For this review, take the finished solid that the model builds, in its own axes (mm). Face numbers are marked on the shaded views. A direction names the side the tool comes from. Round coordinates to 2 decimals unless told otherwise and drop trailing zeros. Loops run counter-clockwise (first coordinate to the right, second up) from the corner with the lowest first, then second, coordinate; pieces in that order, holes last.
1. Clearance check with flat-ended pins moving along their axes: pin 1 Ø4 at (y, z) = (1, 4.5) entering from +X; pin 2 Ø17.5 at (x, z) = (4.5, -0.5) entering from +Y; pin 3 Ø3 at (y, z) = (4, 12) entering from -X. State where each tip first meets the part, or that it passes through.
2. Consider section B-B on z = 0. State the section outline as (x, y) points.
3. To check wall thickness, follow line 1 along Z through (x, y) = (-1.5, 6.75); line 2 along X through (y, z) = (6.5, 6.5); line 3 along X through (y, z) = (7, 6). State the ranges of each line that lie inside material, in increasing order.
4. Consider section C-C on x = 8. State the section outline as (y, z) points, then the cut area to 3 significant figures.
5. Consider section D-D on z = 7.5. State the section outline as (x, y) points.
6. Tool access review of the marked faces 4 and 5: name each direction out of +Z, -Z, +X, -X, +Y, -Y from which nothing blocks a thin tool from reaching the whole face with its end or side.
7. Draft analysis for pull direction Z (two halves, no side actions). For the marked faces 1, 2 and 3, state which applies: released by +Z, released by -Z, zero draft, split by the parting line, or undercut.
8. Consider section A-A on x = 0. State the section outline as (y, z) points, then the cut area to 3 significant figures.
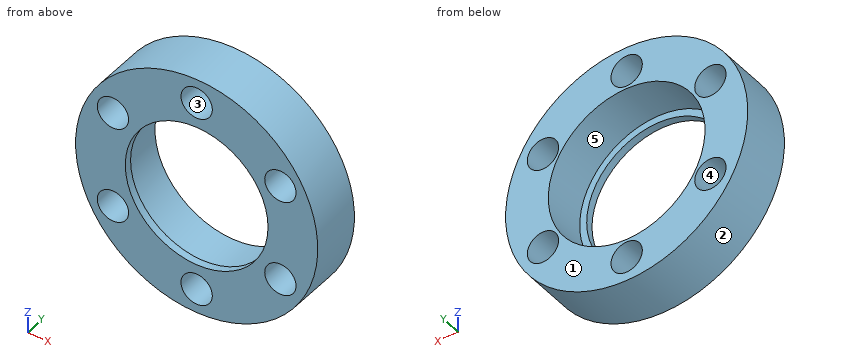
from build123d import *

# Parameters (mm, degrees)
SKETCH1_R         = 16.891
EXTRUDE1_DEPTH    = 7.239
SKETCH2_R         = 10.9347
EXTRUDE2_DEPTH    = 25.960266084
SKETCH3_R         = 10.9347
SKETCH3_R_2       = 9.9568
EXTRUDE3_DEPTH    = 1.0414
SKETCH4_R         = 2.1844
EXTRUDE4_DEPTH    = 25.960266084
CIRPATTERN1_COUNT = 6


with BuildPart() as part:
    # Sketch1 → Extrude1 (new body)
    with BuildSketch(Plane(origin=(0, 0, 0), x_dir=(1, 0, 0), z_dir=(0, 1, 0))):
        with Locations(Location((0, 0, 0), (0, 0, 270))):
            Circle(SKETCH1_R)
    extrude(amount=EXTRUDE1_DEPTH)

    # Sketch2 → Extrude2 (cut, through all)
    with BuildSketch(Plane.XZ):
        with Locations(Location((0, 0, 0), (0, 0, 270))):
            Circle(SKETCH2_R)
    extrude(amount=-EXTRUDE2_DEPTH, mode=Mode.SUBTRACT)

    # Sketch3 → Extrude3 (add)
    with BuildSketch(Plane.XZ):
        with Locations(Location((0, 0, 0), (0, 0, 270))):
            Circle(SKETCH3_R)
        with Locations(Location((0, 0, 0), (0, 0, 270))):
            Circle(SKETCH3_R_2, mode=Mode.SUBTRACT)
    extrude(amount=-EXTRUDE3_DEPTH)

    # Sketch4 → Extrude4 (cut, through all)
    with BuildSketch(Plane(origin=(0, 7.239, 0), x_dir=(1, 0, 0), z_dir=(0, 1, 0))):
        with Locations(Location((0, 13.4874, 0), (0, 0, 270))):
            Circle(SKETCH4_R)
    extrude4 = extrude(amount=-EXTRUDE4_DEPTH, mode=Mode.SUBTRACT)

    # CirPattern1: Extrude4 ×6 about axis
    cirpattern1_axis = Axis((0, 0, 0), (0, 1, 0))
    for i in range(1, CIRPATTERN1_COUNT):
        add(extrude4.rotate(cirpattern1_axis, i * 360 / CIRPATTERN1_COUNT), mode=Mode.SUBTRACT)


solid = part.part
Resolved:
1. pin 1: stops at x = 16.7
1. pin 2: stops at y = 7.24
1. pin 3: stops at x = -13.23
2. outline: (-16.89, 0) - (-9.96, 0) - (-9.96, 1.04) - (-10.93, 1.04) - (-10.93, 7.24) - (-16.89, 7.24) - close; (9.96, 0) - (16.89, 0) - (16.89, 7.24) - (10.93, 7.24) - (10.93, 1.04) - (9.96, 1.04) - close
3. line 1: z = -16.82 to -15.08, -11.9 to -10.83, 10.83 to 11.9, 15.08 to 16.82
3. line 2: x = -15.59 to -13.85, -9.51 to -8.79, 8.79 to 9.51, 13.85 to 15.59
3. line 3: x = -15.79 to -13.73, -9.63 to -9.14, 9.14 to 9.63, 13.73 to 15.79
4. outline: (0, -14.88) - (7.24, -14.88) - (7.24, -7.45) - (1.04, -7.45) - (1.04, -5.93) - (0, -5.93) - close; (0, 5.93) - (1.04, 5.93) - (1.04, 7.45) - (7.24, 7.45) - (7.24, 14.88) - (0, 14.88) - close
4. area: 111 mm2
5. outline: (-15.13, 0) - (-13.73, 0) - (-13.73, 7.24) - (-15.13, 7.24) - close; (-9.63, 0) - (-6.55, 0) - (-6.55, 1.04) - (-7.96, 1.04) - (-7.96, 7.24) - (-9.63, 7.24) - close; (6.55, 0) - (9.63, 0) - (9.63, 7.24) - (7.96, 7.24) - (7.96, 1.04) - (6.55, 1.04) - close; (13.73, 0) - (15.13, 0) - (15.13, 7.24) - (13.73, 7.24) - close
6. face 4: +Y, -Y
6. face 5: +Y
7. face 1: zero draft
7. face 2: split by the parting line
7. face 3: undercut
8. outline: (0, -16.89) - (7.24, -16.89) - (7.24, -15.67) - (0, -15.67) - close; (0, -11.3) - (7.24, -11.3) - (7.24, -10.93) - (1.04, -10.93) - (1.04, -9.96) - (0, -9.96) - close; (0, 9.96) - (1.04, 9.96) - (1.04, 10.93) - (7.24, 10.93) - (7.24, 11.3) - (0, 11.3) - close; (0, 15.67) - (7.24, 15.67) - (7.24, 16.89) - (0, 16.89) - close
8. area: 25.0 mm2
